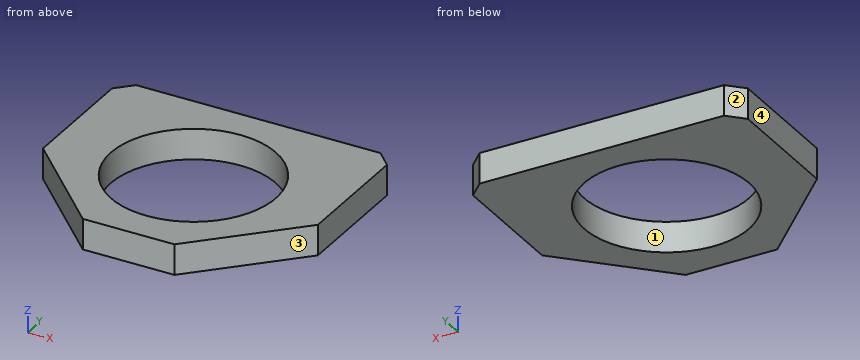
```python
from build123d import *

# Parameters (mm, degrees)
SKETCH1_W                   = 18
SKETCH1_H                   = 15
BOSS_EXTRUDE1_DEPTH         = 2
CHAMFER1_SIZE               = 1
M12X1_25_TAPPED_HOLE1_D     = 10.8
M12X1_25_TAPPED_HOLE1_DEPTH = 8.75
M12X1_25_TAPPED_HOLE1_TIP   = 3.244647343
CHAMFER2_SIZE               = 6


with BuildPart() as part:
    # Sketch1 → Boss-Extrude1 (new body)
    with BuildSketch(Plane.XY):
        Rectangle(SKETCH1_W, SKETCH1_H)
    extrude(amount=BOSS_EXTRUDE1_DEPTH)

    # Chamfer1
    chamfer1_edges = [part.edges().sort_by_distance(p)[0] for p in [
        (-9, 7.5, 1),
        (9, 7.5, 1),
    ]]
    chamfer(chamfer1_edges, length=CHAMFER1_SIZE)

    # M12x1.25 Tapped Hole1
    with Locations(Plane.XY.offset(2)):
        with Locations((0, 0)):
            Hole(M12X1_25_TAPPED_HOLE1_D / 2, depth=M12X1_25_TAPPED_HOLE1_DEPTH)
            with Locations((0, 0, -(M12X1_25_TAPPED_HOLE1_DEPTH + M12X1_25_TAPPED_HOLE1_TIP / 2))):  # 118° drill point
                Cone(0, M12X1_25_TAPPED_HOLE1_D / 2, M12X1_25_TAPPED_HOLE1_TIP, mode=Mode.SUBTRACT)

    # Chamfer2
    chamfer2_edges = [part.edges().sort_by_distance(p)[0] for p in [
        (9, -7.5, 1),
        (-9, -7.5, 1),
    ]]
    chamfer(chamfer2_edges, length=CHAMFER2_SIZE)


solid = part.part
```
CAD build for the part. Positions are in the model's coordinates, mm. Face numbers are marked on the shaded views. Round coordinates to 2 decimals unless told otherwise and drop trailing zeros. Order: outer loops, then holes, each group sorted by start corner. A loop starts at its lowest first (then second) coordinate and runs counter-clockwise, first axis right, second up. Notation, with made-up numbers: (1, 81.5) - (36, 81.5) arc R19 ccw to (36, 110.5) - close; hole circle Ø5 at (84, 88). An arc over 180 degrees is marked (long way). Answer in a Markdown table with one row per item. Add a question column.
(1) Band-saw the part on B-B on x = 0. List the corners of the cut face in (y, z), and give its area (3 significant figures).
(2) Band-saw the part on D-D on y = -6.25. List the corners of the cut face in (x, z), and give its area (3 significant figures).
(3) Probe L1, parallel to Y at x = 0, z = 1.25; L2, parallel to X at y = 0.75, z = 1.3; L3, parallel to X at y = 0.5, z = 1.3. List the from-to ranges inside material, lowest first. Write a range as [from, to].
(4) Band-saw the part on C-C on z = 0.2. List the corners of the cut face in (x, y), and give its area (3 significant figures).
(5) Mould opens along Y. For the marked faces 1, 2, 3 and 4 say: +Y half, -Y half, draft (parallel to the pull), parting line (faces both ways), or undercut.
(6) Drop a flat-ended pin along its axis: pin 1 Ø6 at (x, y) = (-4.5, 5) entering from -Z. Give the stop position or say it passes through.
(7) Band-saw the part on A-A on y = 0. List the corners of the cut face in (x, z), and give its area (3 significant figures).
Data:
| question | item | result |
|---|---|---|
| 1 | outline | (-7.5, 0) - (-5.4, 0) - (-5.4, 2) - (-7.5, 2) - close; (5.4, 0) - (7.5, 0) - (7.5, 2) - (5.4, 2) - close |
| 1 | area | 8.40 mm^2 |
| 2 | outline | (-4.25, 0) - (4.25, 0) - (4.25, 2) - (-4.25, 2) - close |
| 2 | area | 17.0 mm^2 |
| 3 | L1 | y = [-7.5, -5.4], [5.4, 7.5] |
| 3 | L2 | x = [-9, -5.35], [5.35, 9] |
| 3 | L3 | x = [-9, -5.38], [5.38, 9] |
| 4 | outline | (-9, -1.5) - (-3, -7.5) - (3, -7.5) - (9, -1.5) - (9, 6.5) - (8, 7.5) - (-8, 7.5) - (-9, 6.5) - close; hole circle Ø10.8 at (0, 0) |
| 4 | area | 141 mm^2 |
| 5 | face 1 | undercut |
| 5 | face 2 | +Y half |
| 5 | face 3 | -Y half |
| 5 | face 4 | draft |
| 6 | pin 1 | stops at z = 0 |
| 7 | outline | (-9, 0) - (-5.4, 0) - (-5.4, 2) - (-9, 2) - close; (5.4, 0) - (9, 0) - (9, 2) - (5.4, 2) - close |
| 7 | area | 14.4 mm^2 |
